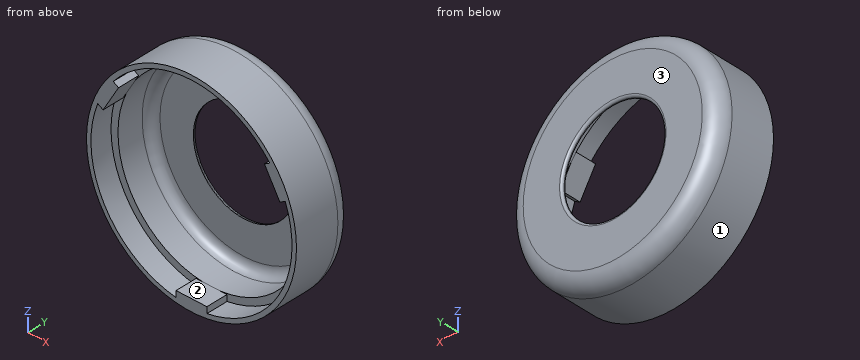
from build123d import *

# Parameters (mm, degrees)
FILLET2_R           = 0.75
BOSS_EXTRUDE4_DEPTH = 7


with BuildPart() as part:
    # Sketch5 → Revolve1 (revolve)
    with BuildSketch(Plane.XY):
        with BuildLine():
            Line((30.3, 7.697016625), (30.3, 16.110174346))
            ThreePointArc((30.3, 16.110174346), (29.421320344, 18.23149469), (27.3, 19.110174346))
            Line((27.3, 19.110174346), (22.498120145, 19.110174346))
            Line((22.498120145, 19.110174346), (16.498120145, 19.110174346))
            Line((16.498120145, 19.110174346), (16.498120145, 20.138377289))
            Line((16.498120145, 20.138377289), (29, 20.138377289))
            ThreePointArc((29, 20.138377289), (32.535533906, 18.673911195), (34, 15.138377289))
            Line((34, 15.138377289), (34, 0.697016625))
            Line((34, 0.697016625), (32.55, 0.697016625))
            Line((32.55, 0.697016625), (32.55, 7.697016625))
            Line((32.55, 7.697016625), (30.3, 7.697016625))
        make_face()
    revolve(axis=Axis((0, 0, 0), (0, 1, 0)))

    # Fillet2
    fillet2_edges = [part.edges().sort_by_distance(p)[0] for p in [
        (-16.498120145, 20.138377289, 0),
    ]]
    fillet(fillet2_edges, radius=FILLET2_R)

    # Sketch8 → Boss-Extrude4 (add)
    with BuildSketch(Plane.XZ.offset(-0.697016625)):
        with BuildLine():
            Line((-5, -30.163682936), (5, -30.163682936))
            Line((5, -30.163682936), (5, -32.163682936))
            ThreePointArc((5, -32.163682936), (0, -32.55), (-5, -32.163682936))
            Line((-5, -32.163682936), (-5, -30.163682936))
        make_face()
        with BuildLine():
            Line((-28.622515694, 10.751714449), (-30.354566502, 11.751714449))
            ThreePointArc((-30.354566502, 11.751714449), (-28.189126893, 16.275), (-25.354566502, 20.411968487))
            Line((-25.354566502, 20.411968487), (-23.622515694, 19.411968487))
            Line((-23.622515694, 19.411968487), (-28.622515694, 10.751714449))
        make_face()
        with BuildLine():
            Line((23.622515694, 19.411968487), (25.354566502, 20.411968487))
            ThreePointArc((25.354566502, 20.411968487), (28.189126893, 16.275), (30.354566502, 11.751714449))
            Line((30.354566502, 11.751714449), (28.622515694, 10.751714449))
            Line((28.622515694, 10.751714449), (23.622515694, 19.411968487))
        make_face()
    extrude(amount=-BOSS_EXTRUDE4_DEPTH)


solid = part.part
Could you check a few things on this model? Use its own coordinates, in mm. Face numbers are marked on the shaded views. Give positions to 0.01 mm unless a question says otherwise; leave off trailing zeros. Order: outer loops, then holes, each group sorted by start corner. A loop starts at its lowest first (then second) coordinate and runs counter-clockwise, first axis right, second up.
1. Suppose I cut it at B-B (x = 0). Write out the boundary of the cut face in (y, z), plus the area to 3 significant figures.
Answers below:
outline: (0.7, -34) - (15.14, -34) arc R5 ccw to (20.14, -29) - (20.14, -17.25) arc R0.75 ccw to (19.39, -16.5) - (19.11, -16.5) - (19.11, -27.3) arc R3 cw to (16.11, -30.3) - (7.7, -30.3) - (7.7, -30.16) - (0.7, -30.16) - close; (0.7, 32.55) - (7.7, 32.55) - (7.7, 30.3) - (16.11, 30.3) arc R3 cw to (19.11, 27.3) - (19.11, 16.5) - (19.39, 16.5) arc R0.75 ccw to (20.14, 17.25) - (20.14, 29) arc R5 ccw to (15.14, 34) - (0.7, 34) - close
area: 150 mm2
2. Suppose I cut it at C-C (z = 0). Write out the boundary of the cut face in (x, y), plus the area to 3 significant figures.
Answers below:
outline: (-34, 0.7) - (-32.55, 0.7) - (-32.55, 7.7) - (-30.3, 7.7) - (-30.3, 16.11) arc R3 cw to (-27.3, 19.11) - (-16.5, 19.11) - (-16.5, 19.39) arc R0.75 ccw to (-17.25, 20.14) - (-29, 20.14) arc R5 ccw to (-34, 15.14) - close; (16.5, 19.11) - (27.3, 19.11) arc R3 cw to (30.3, 16.11) - (30.3, 7.7) - (32.55, 7.7) - (32.55, 0.7) - (34, 0.7) - (34, 15.14) arc R5 ccw to (29, 20.14) - (17.25, 20.14) arc R0.75 ccw to (16.5, 19.39) - close
area: 134 mm2
3. Suppose I cut it at A-A (y = 6). Write out the boundary of the cut face in (x, z), plus the area to 3 significant figures.
Answers below:
outline: circle Ø68 at (0, 0); hole (-30.35, 11.75) arc R32.55 ccw to (-5, -32.16) - (-5, -30.16) - (5, -30.16) - (5, -32.16) arc R32.55 ccw to (30.35, 11.75) - (28.62, 10.75) - (23.62, 19.41) - (25.35, 20.41) arc R32.55 ccw to (-25.35, 20.41) - (-23.62, 19.41) - (-28.62, 10.75) - close
area: 371 mm2
4. Thinking about a two-plate mould opening in Z: for the marked faces 1, 2 and 3, which applies, +Z half, -Z half, draft (parallel to the pull), parting line (faces both ways), or undercut?
Answers below:
face 1: parting line
face 2: undercut
face 3: draft
5. For pin 1 (1.5 mm diameter, centred on y = 18, z = -5, fed in from -X); pin 2 (1.5 mm diameter, centred on x = 15, y = 15.5, fed in from +Z); pin 3 (0.9 mm diameter, centred on x = -26, z = 14.5, fed in from +Y), each with a flat end and sliding along its axis, tell me the tip position at first contact or that it passes through.
Answers below:
pin 1: stops at x = -33.17
pin 2: stops at z = 30.86
pin 3: stops at y = 20.13
6. I need wall thicknesses on L1, parallel to Z at x = 0, y = 10; L2, parallel to Z at x = -25, y = 7.25; L3, parallel to Y at x = -24, z = -10.5. Which ranges of each line are inside material? Lowest first, please.
Answers below:
L1: z = -34 to -30.3, 30.3 to 34
L2: z = -23.04 to -20.84, 17.03 to 20.21, 20.84 to 23.04
L3: y = 19.11 to 20.14
